Design review of the part built by this model. Coordinates are the model's own, in mm. Coordinates: 2 decimals unless noted, no trailing zeros. Order: outer loops, then holes, each group sorted by start corner. A loop starts at its lowest first (then second) coordinate and runs counter-clockwise, first axis right, second up. Notation, with made-up numbers: (77.5, 37) - (106.5, 37) arc R13 cw to (106.5, 49) - close; hole circle Ø5 at (72, 72.5). An arc over 180 degrees is marked (long way). Write each question's results on one line, items separated by ' | '. Start each with the question number.
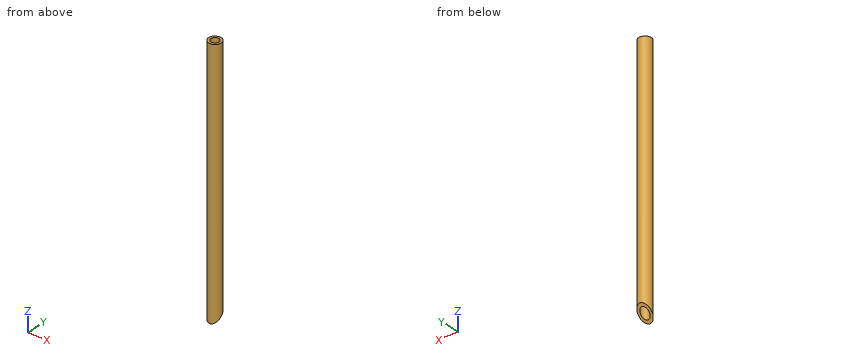
```python
from build123d import *

# Parameters (mm, degrees)
F0_R     = 3
F1_DEPTH = 130
F2_T     = -1.1
F5_R     = 26.2587558367
F6_DEPTH = 25


with BuildPart() as f1:
    # F0 (on Top) → F1 (new body)
    with BuildSketch(Plane.XY):
        Circle(F0_R)
    extrude(amount=F1_DEPTH)

    # F2
    f2_openings = [f1.faces().sort_by_distance(p)[0] for p in [
        (0, 0, 130),
    ]]
    offset(amount=F2_T, openings=f2_openings)

    # F5 (on face) → F6 (cut)
    with BuildSketch(Plane(origin=(0, -7.0710678119, 7.0710678119), x_dir=(1, 0, 0), z_dir=(0, -0.7071067812, 0.7071067812))):
        Circle(F5_R)
    extrude(amount=-F6_DEPTH, mode=Mode.SUBTRACT)


solid = f1.part
```
(1) Clearance check with flat-ended pins moving along their axes: pin 1 (1.5 mm diameter, centred on x = -2.5, y = -0.5, fed in from -Z); pin 2 (1.5 mm diameter, centred on x = -1.5, z = 71, fed in from -Y); pin 3 (1.5 mm diameter, centred on y = 2, z = 35.5, fed in from +X); pin 4 (1 mm diameter, centred on x = -0.5, z = 104, fed in from -Y). State where each tip first meets the part, or that it passes through.
(2) To check wall thickness, follow line 1 along Y through (x, z) = (0, 62); line 2 along Z through (x, y) = (1.55, -1.9). State the ranges of each line that lie inside material, in increasing order. Write a range as [from, to].
(3) Take a section at A-A (x = 0). State the section outline as (y, z) points.
(4) Take a section at C-C (z = 121.5). State the section outline as (x, y) points, plus the area to 3 significant figures.
(5) Take a section at B-B (y = 0). State the section outline as (x, z) points, plus the area to 3 significant figures.
Worked out:
1) pin 1: z = 12.89 | pin 2: y = -2.9 | pin 3: x = 2.73 | pin 4: y = -3
2) line 1: [-3, -1.9], [1.9, 3] | line 2: [12.24, 130]
3) outline: (-3, 11.14) - (-1.9, 12.24) - (-1.9, 130) - (-3, 130) - close; (1.9, 16.04) - (3, 17.14) - (3, 130) - (1.9, 130) - close
4) outline: circle Ø6 at (0, 0); hole circle Ø3.8 at (0, 0) | area: 16.9 mm^2
5) outline: (-3, 14.14) - (-1.9, 14.14) - (-1.9, 130) - (-3, 130) - close; (1.9, 14.14) - (3, 14.14) - (3, 130) - (1.9, 130) - close | area: 255 mm^2
